The model under review builds one solid part; all positions refer to its coordinate system, in mm. Face numbers are marked on the shaded views. A direction names the side the tool comes from. Round coordinates to 2 decimals unless told otherwise and drop trailing zeros. Loops run counter-clockwise (first coordinate to the right, second up) from the corner with the lowest first, then second, coordinate; pieces in that order, holes last. Notation, with made-up numbers: M 49.5,-18 L 107.5,-18 A14 ccw 107.5,1 Z; hole C 78,37 d7. An arc over 180 degrees is marked long. Answer as a JSON object with one key per item and string values. Group by question number.
Item 1: Consider section C-C (y = -1). Give the boundary of the cut face in (x, z) (3 decimals).
Item 2: Tool access review of the marked faces 1 and 2: name each direction out of +Z, -Z, +X, -X, +Y, -Y from which nothing blocks a thin tool from reaching the whole face with its end or side.
Item 3: To check wall thickness, follow line 1 (X direction, y = 8, z = 20.25) (3 decimals); line 2 (Y direction, x = 20.5, z = 2.75) (3 decimals); line 3 (X direction, y = -7, z = 14.75) (3 decimals). State the ranges of each line that lie inside material, in increasing order.
Item 4: Insertion check: P1, Ø5, axis at x = -1, z = 22, coming from the -Y side; P2, Ø5, axis at x = 11, z = 10.5, coming from the -Y side; P3, Ø1, axis at x = -24, z = 9.5, coming from the +Y side (3 decimals). Each pin has a flat end and moves straight along its axis. Give the tip position at first contact, or say it passes through.
Item 5: Consider section B-B (x = -11.5). Give the boundary of the cut face in (y, z) (3 decimals), and give its area (3 significant figures).
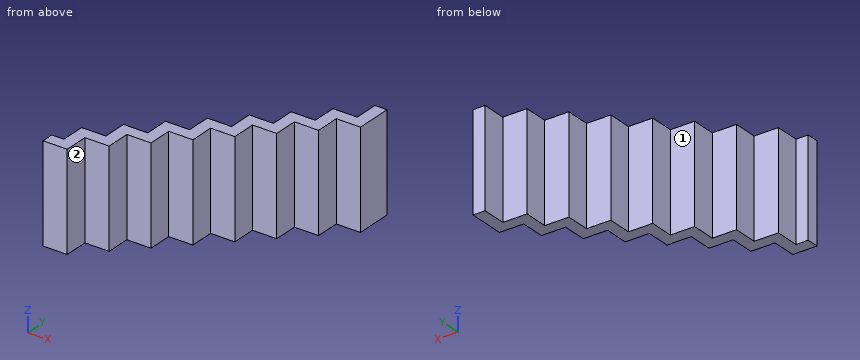
```python
from build123d import *

# Parameters (mm, degrees)
F0_W     = 3.175
F0_H     = 6.35
F1_DEPTH = 25.4


with BuildPart() as f1:
    # F0 (on Top) → F1 (new body)
    with BuildSketch(Plane.XY):
        Polygon((-12.7, -12.7), (-12.7, -9.525), (-15.875, -9.525), (-15.875, -15.875), (-12.7, -15.875), align=None)
        Polygon((-19.05, -19.05), (-19.05, -15.875), (-22.225, -15.875), (-22.225, -22.225), (-19.05, -22.225), align=None)
        Polygon((-12.7, -19.05), (-12.7, -15.875), (-15.875, -15.875), (-19.05, -15.875), (-19.05, -19.05), align=None)
        Polygon((0, -3.175), (0, 0), (0, 3.175), (-3.175, 3.175), (-3.175, -3.175), align=None)
        Polygon((0, -6.35), (0, -3.175), (-3.175, -3.175), (-6.35, -3.175), (-6.35, -6.35), align=None)
        Polygon((-6.35, -6.35), (-6.35, -3.175), (-9.525, -3.175), (-9.525, -9.525), (-6.35, -9.525), align=None)
        Polygon((19.05, 22.225), (19.05, 19.05), (25.4, 19.05), (25.4, 22.225), (22.225, 22.225), align=None)
        Polygon((12.7, 15.875), (12.7, 12.7), (19.05, 12.7), (19.05, 15.875), (15.875, 15.875), align=None)
        Polygon((15.875, 22.225), (15.875, 15.875), (19.05, 15.875), (19.05, 19.05), (19.05, 22.225), align=None)
        Polygon((9.525, 15.875), (9.525, 9.525), (12.7, 9.525), (12.7, 12.7), (12.7, 15.875), align=None)
        Polygon((6.35, 9.525), (6.35, 6.35), (12.7, 6.35), (12.7, 9.525), (9.525, 9.525), align=None)
        Polygon((-6.35, -12.7), (-6.35, -9.525), (-9.525, -9.525), (-12.7, -9.525), (-12.7, -12.7), align=None)
        Polygon((3.175, 3.175), (6.35, 3.175), (6.35, 6.35), (6.35, 9.525), (3.175, 9.525), align=None)
        Polygon((0, 3.175), (0, 0), (6.35, 0), (6.35, 3.175), (3.175, 3.175), align=None)
        Polygon((-19.05, -25.4), (-19.05, -22.225), (-22.225, -22.225), (-25.4, -22.225), (-25.4, -25.4), align=None)
        with Locations((23.8125, 25.4)):
            Rectangle(F0_W, F0_H)
    extrude(amount=F1_DEPTH)


solid = f1.part
```
Geometry results:
{
 "1": {"outline": "M -3.175,0 L 0,0 L 0,25.4 L -3.175,25.4 Z"},
 "2": {"face 1": "+Z, -Z, -X, +Y", "face 2": "+Z, -Z, +X, -Y"},
 "3": {"line 1": "x = 3.175 to 12.7", "line 2": "y = 19.05 to 22.225", "line 3": "x = -9.525 to -6.35"},
 "4": {"P1": "stops at y = -6.35", "P2": "stops at y = 6.35", "P3": "stops at y = -22.225"},
 "5": {"outline": "M -12.7,0 L -9.525,0 L -9.525,25.4 L -12.7,25.4 Z", "area": "80.6 mm^2"}
}
